Model file for the job. Use its own axes, mm. A direction names the side the tool comes from. Round coordinates to 2 decimals unless told otherwise and drop trailing zeros. Order: outer loops, then holes, each group sorted by start corner. A loop starts at its lowest first (then second) coordinate and runs counter-clockwise, first axis right, second up. Notation, with made-up numbers: (-21, 66) - (11, 66) arc R25 cw to (11, 89) - close; hole circle Ø8 at (19, 57). An arc over 180 degrees is marked (long way). Write item = value, one per line.
```python
from build123d import *

# Parameters (mm, degrees)
F0_W      = 123
F0_H      = 100
F0_R      = 2
F1_DEPTH  = 3
F2_W      = 3
F2_H      = 100
F3_DEPTH  = 50
F4_W      = 120
F4_H      = 3
F5_DEPTH  = 50
F6_R      = 2
F7_DEPTH  = 53.001
F8_R      = 2
F9_DEPTH  = 123.001
F10_W     = 3
F10_H     = 50
F11_DEPTH = 10
F13_DEPTH = 10


with BuildPart() as f1:
    # F0 (on Front) → F1 (new body)
    with BuildSketch(Plane.XZ):
        with Locations((61.5, -50)):
            Rectangle(F0_W, F0_H)
        with Locations((34, -90)):
            Circle(F0_R, mode=Mode.SUBTRACT)
        Polygon((10, -82), (10, -58), (52, -58), (58, -64), (58, -76), (52, -82), align=None, mode=Mode.SUBTRACT)
        with Locations((34, -50)):
            Circle(F0_R, mode=Mode.SUBTRACT)
    extrude(amount=F1_DEPTH)

    # F2 (on face) → F3 (join)
    with BuildSketch(Plane(origin=(0, 0, 0), x_dir=(-1, 0, 0), z_dir=(0, 1, 0))):
        with Locations((-121.5, -50)):
            Rectangle(F2_W, F2_H)
    extrude(amount=F3_DEPTH)

    # F4 (on face) → F5 (join)
    with BuildSketch(Plane(origin=(0, 0, 0), x_dir=(-1, 0, 0), z_dir=(0, 1, 0))):
        with Locations((-60, -98.5)):
            Rectangle(F4_W, F4_H)
    extrude(amount=F5_DEPTH)

    # F6 (on face) → F7 (cut, through all)
    with BuildSketch(Plane.XZ.offset(3)):
        with Locations((20, -10)):
            Circle(F6_R)
    extrude(amount=-F7_DEPTH, mode=Mode.SUBTRACT)

    # F8 (on face) → F9 (cut, through all)
    with BuildSketch(Plane.YZ.offset(123)):
        with Locations((25, -10)):
            Circle(F8_R)
    extrude(amount=-F9_DEPTH, mode=Mode.SUBTRACT)

    # F10 (on face) → F11 (join)
    with BuildSketch(Plane.XY.offset(-97)):
        with Locations((1.5, 25)):
            Rectangle(F10_W, F10_H)
    extrude(amount=F11_DEPTH)

    # F12 (on face) → F13 (join)
    with BuildSketch(Plane(origin=(0, 50, 0), x_dir=(-1, 0, 0), z_dir=(0, 1, 0))):
        Polygon((-120, -35), (-120, -50), (-114, -39.607695), (-114, -28), (-117, -28), (-117, -35), align=None)
    extrude(amount=-F13_DEPTH)


solid = f1.part
```
1) Cut at A-A (x = 20). Write the cut outline in (y, z).
Conclusion:
outline = (-3, -100) - (50, -100) - (50, -97) - (0, -97) - (0, -82) - (-3, -82) - close; (-3, -58) - (0, -58) - (0, -12) - (-3, -12) - close; (-3, -8) - (0, -8) - (0, 0) - (-3, 0) - close
2) Cut at B-B (z = -90). Write the cut outline in (x, y), and give its area (3 significant figures).
Conclusion:
outline = (0, -3) - (32, -3) - (32, 0) - (3, 0) - (3, 50) - (0, 50) - close; (36, -3) - (123, -3) - (123, 50) - (120, 50) - (120, 0) - (36, 0) - close
area = 657 mm^2
3) Mould opens along Y. For faces 5 (the face through (55, -1, -61)), 6 (the face through (117, 40, -39)), 7 (the face through (89, 50, -98)) say: +Y half, -Y half, draft (parallel to the pull), parting line (faces both ways), or undercut.
Conclusion:
face_5 = draft
face_6 = undercut
face_7 = +Y half
4) Cut at D-D (y = 13.5). Write the cut outline in (x, z), and give its area (3 significant figures).
Conclusion:
outline = (0, -100) - (123, -100) - (123, 0) - (120, 0) - (120, -97) - (3, -97) - (3, -87) - (0, -87) - close
area = 690 mm^2
5) 3-axis set-ups, long thin cutter, end or side, ignore diameter. For faces 1 (the face through (117.042, 45.07, -44.877)), 2 (the face through (55, -1, -79)), 3 (the face through (117, 45, -31)), 4 (the face through (62, 23, -100)): which of +Z, -Z, +X, -X, +Y, -Y reach the whole face in a straight line?
Conclusion:
face_1 = -X, +Y
face_2 = +Y, -Y
face_3 = +Z, +Y
face_4 = -Z, +X, -X, +Y, -Y
6) Wall check: line 1 along Z through (x, y) = (34, -1.45); line 2 along Z through (x, y) = (121.45, 25); line 3 along X through (y, z) = (2, -90). Give the ranges that are in metal, low to high.
Conclusion:
line_1 = -100 to -92, -88 to -82, -58 to -52, -48 to 0
line_2 = -100 to -12, -8 to 0
line_3 = 0 to 3, 120 to 123
7) Flat gauge pins, fed straight in: pin 1 Ø2 at (y, z) = (29, -63.5) entering from -X; pin 2 Ø1.5 at (x, y) = (25, -1.5) entering from +Z; pin 3 Ø11 at (y, z) = (47, -32.5) entering from -X; pin 4 Ø25 at (x, y) = (88, 16) entering from +Z. Where does each tip first touch, or does it go through?
Conclusion:
pin_1 = 120
pin_2 = 0
pin_3 = 114
pin_4 = -97
8) Cut at C-C (x = 39.5). Write the cut outline in (y, z).
Conclusion:
outline = (-3, -100) - (50, -100) - (50, -97) - (0, -97) - (0, -82) - (-3, -82) - close; (-3, -58) - (0, -58) - (0, 0) - (-3, 0) - close
